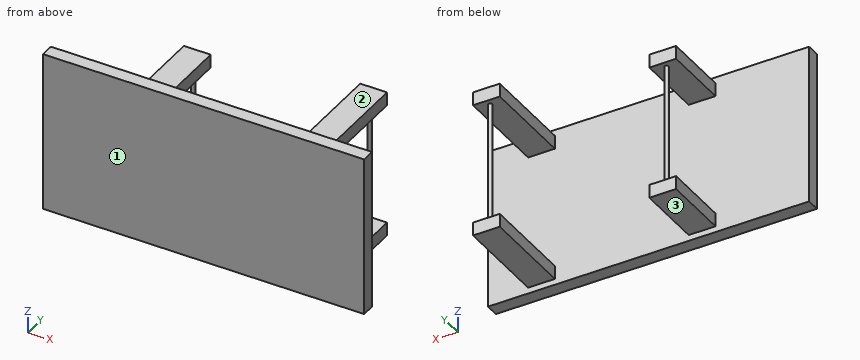
```python
from build123d import *

# Parameters (mm, degrees)
CROQUIS1_W              = 240
CROQUIS1_H              = 120
SALIENTE_EXTRUIR1_DEPTH = 10
CROQUIS2_W              = 20
CROQUIS2_H              = 10
SALIENTE_EXTRUIR2_DEPTH = 50
CROQUIS2_3_W            = 20
CROQUIS2_3_H            = 10
SALIENTE_EXTRUIR3_DEPTH = 70
CROQUIS3_R              = 1.5
SALIENTE_EXTRUIR4_DEPTH = 111


with BuildPart() as part:
    # Croquis1 → Saliente-Extruir1 (new body)
    with BuildSketch(Plane(origin=(0, 0, 0), x_dir=(1, 0, 0), z_dir=(0, 1, 0))):
        Rectangle(CROQUIS1_W, CROQUIS1_H)
    extrude(amount=SALIENTE_EXTRUIR1_DEPTH)

    # Croquis2 → Saliente-Extruir2 (add)
    with BuildSketch(Plane(origin=(0, 10, 0), x_dir=(1, 0, 0), z_dir=(0, 1, 0))):
        with Locations((-40, 50.5)):
            Rectangle(CROQUIS2_W, CROQUIS2_H)
        with Locations((-40, -50.5)):
            Rectangle(CROQUIS2_W, CROQUIS2_H)
    extrude(amount=SALIENTE_EXTRUIR2_DEPTH)

    # Croquis2<3> → Saliente-Extruir3 (add)
    with BuildSketch(Plane(origin=(0, 10, 0), x_dir=(1, 0, 0), z_dir=(0, 1, 0))):
        with Locations((80, 50.5)):
            Rectangle(CROQUIS2_3_W, CROQUIS2_3_H)
        with Locations((80, -50.5)):
            Rectangle(CROQUIS2_3_W, CROQUIS2_3_H)
    extrude(amount=SALIENTE_EXTRUIR3_DEPTH)

    # Croquis3 → Saliente-Extruir4 (add)
    with BuildSketch(Plane.XY.offset(55.5)):
        with Locations((-40, 55)):
            Circle(CROQUIS3_R)
        with Locations((80, 75)):
            Circle(CROQUIS3_R)
    extrude(amount=-SALIENTE_EXTRUIR4_DEPTH)


solid = part.part
```
Geometry: final body of the model. Coordinates: model frame, mm. Face numbers are marked on the shaded views. A direction names the side the tool comes from. Round coordinates to 2 decimals unless told otherwise and drop trailing zeros. Write each loop counter-clockwise with the first axis right and the second up, starting at its lowest first coordinate (ties: lowest second). Pieces come first, ordered by that corner, then holes. Notation, with made-up numbers: M -10.5,70 L 48.5,70 A23 ccw 48.5,108 Z; hole C 45.25,44.5 d2. An arc over 180 degrees is marked long. Answer in a Markdown table with one row per item. Add a question column.
(1) Cut plane B-B, the plane z = -12.5. Return the cut outline in (x, y).
(2) Reachability of the marked faces 1, 2 and 3 from +Z, -Z, +X, -X, +Y, -Y: full face, straight path, thin tool, end or side. Return the list, or none.
(3) Ray query, L1, parallel to X at y = 50.5, z = 55; L2, parallel to Z at x = 70.5, y = 37; L3, parallel to Y at x = -58, z = 37.5. Return the intervals inside material, ascending.
(4) Contact query for flat-ended pins moving along their axis: pin 1 (22 mm diameter, centred on x = -37, y = 24.5, fed in from -Z); pin 2 (3 mm diameter, centred on x = 40.5, z = -35.5, fed in from -Y); pin 3 (8 mm diameter, centred on x = -36, z = 52, fed in from +Y); pin 4 (6 mm diameter, centred on x = 79, y = 46, fed in from +Z). Output: stop coordinate, or through.
(5) Cut plane D-D, the plane x = -103.5. Return the cut outline in (y, z), then the cut area to 3 significant figures.
(6) Cut plane C-C, the plane y = 68. Return the cut outline in (x, z), then the cut area to 3 significant figures.
(7) Cut plane A-A, the plane y = 50. Return the cut outline in (x, z).
Established:
| question | item | result |
|---|---|---|
| 1 | outline | M -120,0 L 120,0 L 120,10 L -120,10 Z; C -40,55 d3; C 80,75 d3 |
| 2 | face 1 | +Z, -Z, +X, -X, -Y |
| 2 | face 2 | +Z, +X, -X, +Y |
| 2 | face 3 | -Z, +X, -X, +Y |
| 3 | L1 | -50 to -30, 70 to 90 |
| 3 | L2 | -55.5 to -45.5, 45.5 to 55.5 |
| 3 | L3 | 0 to 10 |
| 4 | pin 1 | z = -55.5 |
| 4 | pin 2 | y = 0 |
| 4 | pin 3 | y = 60 |
| 4 | pin 4 | z = 55.5 |
| 5 | outline | M 0,-60 L 10,-60 L 10,60 L 0,60 Z |
| 5 | area | 1,200 mm² |
| 6 | outline | M 70,-55.5 L 90,-55.5 L 90,-45.5 L 70,-45.5 Z; M 70,45.5 L 90,45.5 L 90,55.5 L 70,55.5 Z |
| 6 | area | 400 mm² |
| 7 | outline | M -50,-55.5 L -30,-55.5 L -30,-45.5 L -50,-45.5 Z; M -50,45.5 L -30,45.5 L -30,55.5 L -50,55.5 Z; M 70,-55.5 L 90,-55.5 L 90,-45.5 L 70,-45.5 Z; M 70,45.5 L 90,45.5 L 90,55.5 L 70,55.5 Z |
